Source: CAD feature listing. Evaluate the final solid. Frame: model axes, mm. Round coordinates to 2 decimals unless told otherwise and drop trailing zeros. Order: outer loops, then holes, each group sorted by start corner. A loop starts at its lowest first (then second) coordinate and runs counter-clockwise, first axis right, second up. Notation, with made-up numbers: (54.5, -6) -> (92.5, -6) arc R15 ccw to (92.5, 4) -> close; hole circle Ø9 at (5, -28). An arc over 180 degrees is marked (long way). Write item = value, one per line. Start each with the question number.
(1) Ray query, line 1 (Y direction, x = -15, z = -331.5); line 2 (Y direction, x = -12.5, z = -597); line 3 (Y direction, x = -1.5, z = -97.5). Return the intervals inside material, ascending.
(2) Contact query for flat-ended pins moving along their axis: pin 1 Ø1.3 at (y, z) = (74.5, -413.5) entering from +X; pin 2 Ø12 at (x, z) = (-29, -617.5) entering from -Y; pin 3 Ø4 at (y, z) = (75.5, -479.5) entering from -X. Output: stop coordinate, or through.
(3) Cut plane A-A on y = 32.5. Return the cut outline in (x, z), then the cut area to 3 significant figures.
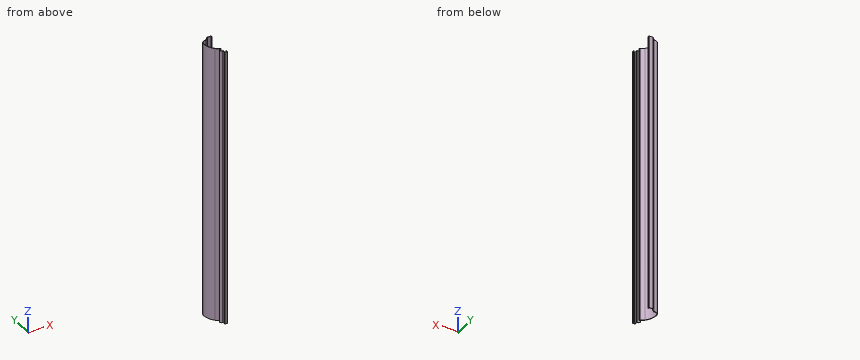
from build123d import *

# Parameters (mm, degrees)
EXTRUDE_THIN1_DEPTH = 920.75
FILLET1_R           = 1.27


with BuildPart() as part:
    # Sketch3 → Extrude-Thin1 (new body)
    with BuildSketch(Plane.XY):
        with BuildLine():
            Line((0, 78.978125), (0, 85.328125))
            Line((0, 85.328125), (-14.2875, 85.328125))
            ThreePointArc((-14.2875, 85.328125), (-16.844823917, 79.154198917), (-23.01875, 76.596875))
            Line((-23.01875, 76.596875), (-23.01875, 74.202381102))
            ThreePointArc((-23.01875, 74.202381102), (-34.102024757, 71.842921697), (-38.889371992, 61.572218972))
            ThreePointArc((-38.889371992, 61.572218972), (-34.427603857, 41.242325722), (-22.75075149, 24.012611469))
            ThreePointArc((-22.75075149, 24.012611469), (-17.030138602, 19.792593223), (-10.31875, 17.449256102))
            Line((-10.31875, 17.449256102), (-10.31875, 15.068006102))
            ThreePointArc((-10.31875, 15.068006102), (-16.665438104, 9.326672958), (-10.715625, 3.175))
            Line((-10.715625, 3.175), (-8.73125, 3.175))
            Line((-8.73125, 3.175), (-8.73125, -6.746875))
            Line((-8.73125, -6.746875), (0, -6.746875))
            Line((0, -6.746875), (0, 0))
            Line((0, 0), (-1.27, 0))
            Line((-1.27, 0), (-1.27, -5.476875))
            Line((-1.27, -5.476875), (-7.46125, -5.476875))
            Line((-7.46125, -5.476875), (-7.46125, 4.445))
            Line((-7.46125, 4.445), (-10.715625, 4.445))
            ThreePointArc((-10.715625, 4.445), (-15.321439486, 9.975552095), (-9.04875, 13.504560479))
            Line((-9.04875, 13.504560479), (-9.04875, 18.527286753))
            ThreePointArc((-9.04875, 18.527286753), (-15.97058408, 20.676234022), (-21.852725878, 24.910637081))
            ThreePointArc((-21.852725878, 24.910637081), (-33.260758622, 41.743696042), (-37.619809793, 61.605562972))
            ThreePointArc((-37.619809793, 61.605562972), (-32.636426474, 71.346888762), (-21.74875, 72.435942687))
            Line((-21.74875, 72.435942687), (-21.74875, 75.407837627))
            ThreePointArc((-21.74875, 75.407837627), (-15.946798305, 78.256173305), (-13.098462627, 84.058125))
            Line((-13.098462627, 84.058125), (-1.27, 84.058125))
            Line((-1.27, 84.058125), (-1.27, 78.978125))
            Line((-1.27, 78.978125), (0, 78.978125))
        make_face()
    extrude(amount=-EXTRUDE_THIN1_DEPTH)

    # Fillet1
    fillet1_edges = [part.edges().sort_by_distance(p)[0] for p in [
        (0, -6.746875, -460.375),
        (-8.73125, -6.746875, -460.375),
        (-23.01875, 76.596875, -460.375),
        (-14.2875, 85.328125, -460.375),
        (0, 85.328125, -460.375),
        (-21.74875, 72.435942687, -460.375),
        (-9.04875, 18.527286753, -460.375),
        (-9.04875, 13.504560479, -460.375),
        (-7.46125, 4.445, -460.375),
    ]]
    fillet(fillet1_edges, radius=FILLET1_R)


solid = part.part
Evaluation:
q1.line_1 = 4.99 to 7.24, 11.02 to 13.26, 18.84 to 20.22, 79.35 to 81.87
q1.line_2 = 3.45 to 4.8, 13.46 to 14.81, 17.97 to 19.29, 84.06 to 85.33
q1.line_3 = -6.75 to -5.48, 84.06 to 85.33
q2.pin_1 = -21.75
q2.pin_2 = 24.26
q2.pin_3 = -31.38
q3.outline = (-29.7, -920.75) -> (-28.16, -920.75) -> (-28.16, 0) -> (-29.7, 0) -> close
q3.area = 1,410 mm^2
